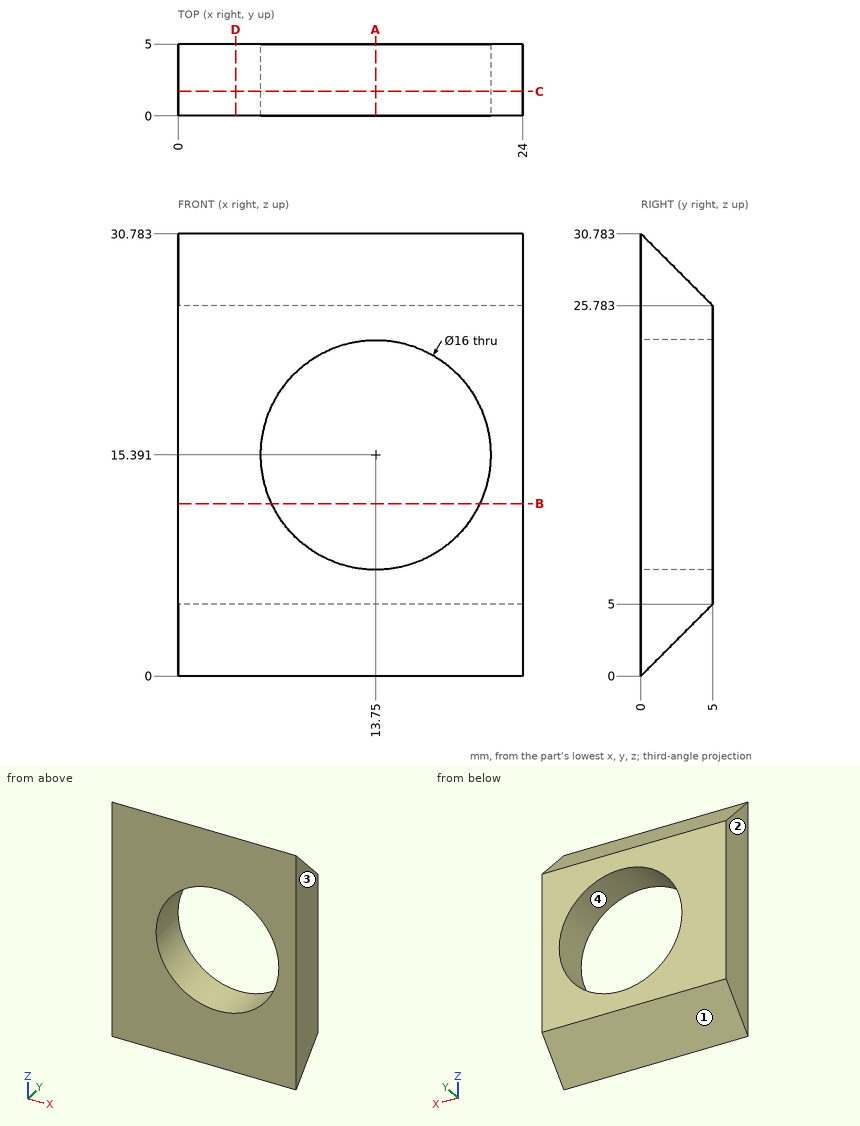
Can you work these out from the drawing? Everything is in mm from the part's minimum corner. Coordinates: 2 decimals unless noted, no trailing zeros. Loops run counter-clockwise (first coordinate to the right, second up) from the corner with the lowest first, then second, coordinate; pieces in that order, holes last.
1) Imagine slicing it at D-D (x = 4). List the corners of the cut face in (y, z) for me, and give its area (3 significant figures).
Reported:
outline: (0, 0) - (5, 5) - (5, 25.78) - (0, 30.78) - close
area: 129 mm2
2) Thinking about a two-plate mould opening in X: for the marked faces 1, 2, 3 and 4, which applies, released by +X, released by -X, zero draft, split by the parting line, or undercut?
Reported:
face 1: zero draft
face 2: released by -X
face 3: released by +X
face 4: undercut
3) Imagine slicing it at B-B (z = 12). List the corners of the cut face in (x, y) for me (1 decimal).
Reported:
outline: (0, 0) - (6.5, 0) - (6.5, 5) - (0, 5) - close; (21, 0) - (24, 0) - (24, 5) - (21, 5) - close
4) Please list where these lines run through material, in increasing order: line 1 along X through (y, z) = (0.85, 15.5); line 2 along X through (y, z) = (1.05, 9); line 3 along Z through (x, y) = (12.5, 4.3) (1 decimal).
Reported:
line 1: x = 0 to 5.75, 21.75 to 24
line 2: x = 0 to 8.94, 18.56 to 24
line 3: z = 4.3 to 7.5, 23.3 to 26.5
5) Will this pin go through, and if not, where does the flat tip stop? pin 1 Ø1.5 at (x, y) = (16.5, 4) entering from +Z.
Reported:
pin 1: stops at z = 27.53
6) Imagine slicing it at C-C (y = 1.7). List the corners of the cut face in (x, z) for me.
Reported:
outline: (0, 1.7) - (24, 1.7) - (24, 29.08) - (0, 29.08) - close; hole circle Ø16 at (13.75, 15.39)
7) Imagine slicing it at A-A (x = 13.75). List the corners of the cut face in (y, z) for me.
Reported:
outline: (0, 0) - (5, 5) - (5, 7.39) - (0, 7.39) - close; (0, 23.39) - (5, 23.39) - (5, 25.78) - (0, 30.78) - close
